The model under review builds one solid part; all positions refer to its coordinate system, in mm. Coordinates: 2 decimals unless noted, no trailing zeros. Loops run counter-clockwise (first coordinate to the right, second up) from the corner with the lowest first, then second, coordinate; pieces in that order, holes last. Notation, with made-up numbers: M 11.5,-16 L 15.5,-16 A16 ccw 15.5,10 Z; hole C 52.25,-17 d10. An arc over 180 degrees is marked long. Use one line per item in the form item = value.
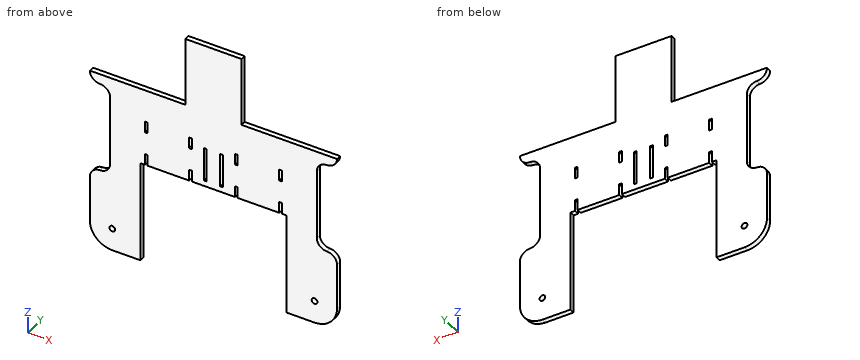
```python
from build123d import *

# Parameters (mm, degrees)
SKETCH1_W           = 279.4
SKETCH1_H           = 279.4
BOSS_EXTRUDE1_DEPTH = 5.715
CUT_EXTRUDE2_REACH  = 199.648
SKETCH4_W           = 22.86
SKETCH4_H           = 101.6
FILLET1_START       = -1
FILLET1_DEPTH       = 8
FILLET1_2_DEPTH     = 5.715
CUT_EXTRUDE3_REACH  = 199.648
SKETCH5_W           = 3.0988
SKETCH5_H           = 12.7
CUT_EXTRUDE4_REACH  = 199.648
SKETCH6_R           = 3.2639
FILLET2_R           = 25.4
CUT_EXTRUDE5_REACH  = 199.648
SKETCH7_W           = 165.1
SKETCH7_H           = 114.3
CUT_EXTRUDE7_REACH  = 199.648
SKETCH16_W          = 3.0988
SKETCH16_H          = 38.1
CUT_EXTRUDE11_REACH = 199.648
SKETCH26_W          = 107.95
SKETCH26_H          = 77.47


with BuildPart() as part:
    # Sketch1 → Boss-Extrude1 (new body)
    with BuildSketch(Plane(origin=(0, 0, 0), x_dir=(1, 0, 0), z_dir=(0, 1, 0))):
        Rectangle(SKETCH1_W, SKETCH1_H)
    extrude(amount=BOSS_EXTRUDE1_DEPTH)

    # Sketch4 → Cut-Extrude2 (cut, up to next)
    with BuildSketch(Plane(origin=(0, 5.715, 0), x_dir=(1, 0, 0), z_dir=(0, 1, 0)), mode=Mode.PRIVATE) as cut_extrude2_sk1:
        with Locations((-128.27, 0)):
            Rectangle(SKETCH4_W, SKETCH4_H)
    cut_extrude2_tool1 = extrude(cut_extrude2_sk1.sketch, amount=-CUT_EXTRUDE2_REACH, mode=Mode.PRIVATE) & part.part
    # Sketch4 → Cut-Extrude2 (cut, up to next)
    with BuildSketch(Plane(origin=(0, 5.715, 0), x_dir=(1, 0, 0), z_dir=(0, 1, 0)), mode=Mode.PRIVATE) as cut_extrude2_sk2:
        with Locations((128.27, 0)):
            Rectangle(SKETCH4_W, SKETCH4_H)
    cut_extrude2_tool2 = extrude(cut_extrude2_sk2.sketch, amount=-CUT_EXTRUDE2_REACH, mode=Mode.PRIVATE) & part.part
    add(cut_extrude2_tool1.solids().sort_by_distance((-128.27, 5.715, 0))[0], mode=Mode.SUBTRACT)
    add(cut_extrude2_tool2.solids().sort_by_distance((128.27, 5.715, 0))[0], mode=Mode.SUBTRACT)

    # Fillet1: read off the stored shape, not the designer's step
    # Fillet1 outline → Fillet1 (cut)
    with BuildSketch(Plane(origin=(0, 0, 0), x_dir=(1, 0, 0), z_dir=(0, 1, 0)).offset(FILLET1_START)):
        with BuildLine():
            ThreePointArc((-139.7, -62.23), (-136.352230509, -54.147769491), (-128.27, -50.8))
            Line((-128.27, -50.8), (-139.7, -50.8))
            Line((-139.7, -50.8), (-139.7, -62.23))
        make_face()
        with BuildLine():
            ThreePointArc((-128.27, 50.8), (-136.352230509, 54.147769491), (-139.7, 62.23))
            Line((-139.7, 62.23), (-139.7, 50.8))
            Line((-139.7, 50.8), (-128.27, 50.8))
        make_face()
        with BuildLine():
            Line((139.7, -50.8), (128.27, -50.8))
            ThreePointArc((128.27, -50.8), (136.352230509, -54.147769491), (139.7, -62.23))
            Line((139.7, -62.23), (139.7, -50.8))
        make_face()
        with BuildLine():
            ThreePointArc((139.7, 62.23), (136.352230509, 54.147769491), (128.27, 50.8))
            Line((128.27, 50.8), (139.7, 50.8))
            Line((139.7, 50.8), (139.7, 62.23))
        make_face()
    extrude(amount=FILLET1_DEPTH, mode=Mode.SUBTRACT)

    # Fillet1 2 outline → Fillet1 2 (add)
    with BuildSketch(Plane(origin=(0, 0, 0), x_dir=(1, 0, 0), z_dir=(0, 1, 0))):
        with BuildLine():
            Line((-116.84, -50.8), (-116.84, -39.37))
            ThreePointArc((-116.84, -39.37), (-120.187769491, -47.452230509), (-128.27, -50.8))
            Line((-128.27, -50.8), (-116.84, -50.8))
        make_face()
        with BuildLine():
            Line((-116.84, 50.8), (-128.27, 50.8))
            ThreePointArc((-128.27, 50.8), (-120.187769491, 47.452230509), (-116.84, 39.37))
            Line((-116.84, 39.37), (-116.84, 50.8))
        make_face()
        with BuildLine():
            Line((116.84, -50.8), (128.27, -50.8))
            ThreePointArc((128.27, -50.8), (120.187769491, -47.452230509), (116.84, -39.37))
            Line((116.84, -39.37), (116.84, -50.8))
        make_face()
        with BuildLine():
            Line((116.84, 50.8), (116.84, 39.37))
            ThreePointArc((116.84, 39.37), (120.187769491, 47.452230509), (128.27, 50.8))
            Line((128.27, 50.8), (116.84, 50.8))
        make_face()
    extrude(amount=FILLET1_2_DEPTH)

    # Sketch5 → Cut-Extrude3 (cut, up to next)
    with BuildSketch(Plane(origin=(0, 0, 0), x_dir=(-1, 0, 0), z_dir=(0, -1, 0)), mode=Mode.PRIVATE) as cut_extrude3_sk1:
        with Locations((75.8825, -19.05)):
            Rectangle(SKETCH5_W, SKETCH5_H)
    cut_extrude3_tool1 = extrude(cut_extrude3_sk1.sketch, amount=-CUT_EXTRUDE3_REACH, mode=Mode.PRIVATE) & part.part
    # Sketch5 → Cut-Extrude3 (cut, up to next)
    with BuildSketch(Plane(origin=(0, 0, 0), x_dir=(-1, 0, 0), z_dir=(0, -1, 0)), mode=Mode.PRIVATE) as cut_extrude3_sk2:
        with Locations((75.8825, 19.05)):
            Rectangle(SKETCH5_W, SKETCH5_H)
    cut_extrude3_tool2 = extrude(cut_extrude3_sk2.sketch, amount=-CUT_EXTRUDE3_REACH, mode=Mode.PRIVATE) & part.part
    # Sketch5 → Cut-Extrude3 (cut, up to next)
    with BuildSketch(Plane(origin=(0, 0, 0), x_dir=(-1, 0, 0), z_dir=(0, -1, 0)), mode=Mode.PRIVATE) as cut_extrude3_sk3:
        with Locations((-75.8825, 19.05)):
            Rectangle(SKETCH5_W, SKETCH5_H)
    cut_extrude3_tool3 = extrude(cut_extrude3_sk3.sketch, amount=-CUT_EXTRUDE3_REACH, mode=Mode.PRIVATE) & part.part
    # Sketch5 → Cut-Extrude3 (cut, up to next)
    with BuildSketch(Plane(origin=(0, 0, 0), x_dir=(-1, 0, 0), z_dir=(0, -1, 0)), mode=Mode.PRIVATE) as cut_extrude3_sk4:
        with Locations((-75.8825, -19.05)):
            Rectangle(SKETCH5_W, SKETCH5_H)
    cut_extrude3_tool4 = extrude(cut_extrude3_sk4.sketch, amount=-CUT_EXTRUDE3_REACH, mode=Mode.PRIVATE) & part.part
    # Sketch5 → Cut-Extrude3 (cut, up to next)
    with BuildSketch(Plane(origin=(0, 0, 0), x_dir=(-1, 0, 0), z_dir=(0, -1, 0)), mode=Mode.PRIVATE) as cut_extrude3_sk5:
        with Locations((25.908, -19.05)):
            Rectangle(SKETCH5_W, SKETCH5_H)
    cut_extrude3_tool5 = extrude(cut_extrude3_sk5.sketch, amount=-CUT_EXTRUDE3_REACH, mode=Mode.PRIVATE) & part.part
    # Sketch5 → Cut-Extrude3 (cut, up to next)
    with BuildSketch(Plane(origin=(0, 0, 0), x_dir=(-1, 0, 0), z_dir=(0, -1, 0)), mode=Mode.PRIVATE) as cut_extrude3_sk6:
        with Locations((25.908, 19.05)):
            Rectangle(SKETCH5_W, SKETCH5_H)
    cut_extrude3_tool6 = extrude(cut_extrude3_sk6.sketch, amount=-CUT_EXTRUDE3_REACH, mode=Mode.PRIVATE) & part.part
    # Sketch5 → Cut-Extrude3 (cut, up to next)
    with BuildSketch(Plane(origin=(0, 0, 0), x_dir=(-1, 0, 0), z_dir=(0, -1, 0)), mode=Mode.PRIVATE) as cut_extrude3_sk7:
        with Locations((-25.908, 19.05)):
            Rectangle(SKETCH5_W, SKETCH5_H)
    cut_extrude3_tool7 = extrude(cut_extrude3_sk7.sketch, amount=-CUT_EXTRUDE3_REACH, mode=Mode.PRIVATE) & part.part
    # Sketch5 → Cut-Extrude3 (cut, up to next)
    with BuildSketch(Plane(origin=(0, 0, 0), x_dir=(-1, 0, 0), z_dir=(0, -1, 0)), mode=Mode.PRIVATE) as cut_extrude3_sk8:
        with Locations((-25.908, -19.05)):
            Rectangle(SKETCH5_W, SKETCH5_H)
    cut_extrude3_tool8 = extrude(cut_extrude3_sk8.sketch, amount=-CUT_EXTRUDE3_REACH, mode=Mode.PRIVATE) & part.part
    add(cut_extrude3_tool1.solids().sort_by_distance((-75.8825, 0, 19.05))[0], mode=Mode.SUBTRACT)
    add(cut_extrude3_tool2.solids().sort_by_distance((-75.8825, 0, -19.05))[0], mode=Mode.SUBTRACT)
    add(cut_extrude3_tool3.solids().sort_by_distance((75.8825, 0, -19.05))[0], mode=Mode.SUBTRACT)
    add(cut_extrude3_tool4.solids().sort_by_distance((75.8825, 0, 19.05))[0], mode=Mode.SUBTRACT)
    add(cut_extrude3_tool5.solids().sort_by_distance((-25.908, 0, 19.05))[0], mode=Mode.SUBTRACT)
    add(cut_extrude3_tool6.solids().sort_by_distance((-25.908, 0, -19.05))[0], mode=Mode.SUBTRACT)
    add(cut_extrude3_tool7.solids().sort_by_distance((25.908, 0, -19.05))[0], mode=Mode.SUBTRACT)
    add(cut_extrude3_tool8.solids().sort_by_distance((25.908, 0, 19.05))[0], mode=Mode.SUBTRACT)

    # Sketch6 → Cut-Extrude4 (cut, up to next)
    with BuildSketch(Plane(origin=(0, 5.715, 0), x_dir=(1, 0, 0), z_dir=(0, 1, 0)), mode=Mode.PRIVATE) as cut_extrude4_sk1:
        with Locations(Location((-114.3, 114.3, 0), (0, 0, 270))):
            Circle(SKETCH6_R)
    cut_extrude4_tool1 = extrude(cut_extrude4_sk1.sketch, amount=-CUT_EXTRUDE4_REACH, mode=Mode.PRIVATE) & part.part
    # Sketch6 → Cut-Extrude4 (cut, up to next)
    with BuildSketch(Plane(origin=(0, 5.715, 0), x_dir=(1, 0, 0), z_dir=(0, 1, 0)), mode=Mode.PRIVATE) as cut_extrude4_sk2:
        with Locations(Location((114.3, 114.3, 0), (0, 0, 270))):
            Circle(SKETCH6_R)
    cut_extrude4_tool2 = extrude(cut_extrude4_sk2.sketch, amount=-CUT_EXTRUDE4_REACH, mode=Mode.PRIVATE) & part.part
    # Sketch6 → Cut-Extrude4 (cut, up to next)
    with BuildSketch(Plane(origin=(0, 5.715, 0), x_dir=(1, 0, 0), z_dir=(0, 1, 0)), mode=Mode.PRIVATE) as cut_extrude4_sk3:
        with Locations(Location((114.3, -114.3, 0), (0, 0, 270))):
            Circle(SKETCH6_R)
    cut_extrude4_tool3 = extrude(cut_extrude4_sk3.sketch, amount=-CUT_EXTRUDE4_REACH, mode=Mode.PRIVATE) & part.part
    # Sketch6 → Cut-Extrude4 (cut, up to next)
    with BuildSketch(Plane(origin=(0, 5.715, 0), x_dir=(1, 0, 0), z_dir=(0, 1, 0)), mode=Mode.PRIVATE) as cut_extrude4_sk4:
        with Locations(Location((-114.3, -114.3, 0), (0, 0, 270))):
            Circle(SKETCH6_R)
    cut_extrude4_tool4 = extrude(cut_extrude4_sk4.sketch, amount=-CUT_EXTRUDE4_REACH, mode=Mode.PRIVATE) & part.part
    add(cut_extrude4_tool1.solids().sort_by_distance((-114.3, 5.715, -114.3))[0], mode=Mode.SUBTRACT)
    add(cut_extrude4_tool2.solids().sort_by_distance((114.3, 5.715, -114.3))[0], mode=Mode.SUBTRACT)
    add(cut_extrude4_tool3.solids().sort_by_distance((114.3, 5.715, 114.3))[0], mode=Mode.SUBTRACT)
    add(cut_extrude4_tool4.solids().sort_by_distance((-114.3, 5.715, 114.3))[0], mode=Mode.SUBTRACT)

    # Fillet2
    fillet2_edges = [part.edges().sort_by_distance(p)[0] for p in [
        (-139.7, 2.8575, -139.7),
        (139.7, 2.8575, -139.7),
        (139.7, 2.8575, 139.7),
        (-139.7, 2.8575, 139.7),
    ]]
    fillet(fillet2_edges, radius=FILLET2_R)

    # Sketch7 → Cut-Extrude5 (cut, up to next)
    with BuildSketch(Plane(origin=(0, 5.715, 0), x_dir=(1, 0, 0), z_dir=(0, 1, 0)), mode=Mode.PRIVATE) as cut_extrude5_sk1:
        with Locations((0, 82.55)):
            Rectangle(SKETCH7_W, SKETCH7_H)
    cut_extrude5_tool1 = extrude(cut_extrude5_sk1.sketch, amount=-CUT_EXTRUDE5_REACH, mode=Mode.PRIVATE) & part.part
    add(cut_extrude5_tool1.solids().sort_by_distance((0, 5.715, -82.55))[0], mode=Mode.SUBTRACT)

    # Sketch16 → Cut-Extrude7 (cut, up to next)
    with BuildSketch(Plane(origin=(0, 5.715, 0), x_dir=(1, 0, 0), z_dir=(0, 1, 0)), mode=Mode.PRIVATE) as cut_extrude7_sk1:
        with Locations((-9.1948, 0)):
            Rectangle(SKETCH16_W, SKETCH16_H)
    cut_extrude7_tool1 = extrude(cut_extrude7_sk1.sketch, amount=-CUT_EXTRUDE7_REACH, mode=Mode.PRIVATE) & part.part
    # Sketch16 → Cut-Extrude7 (cut, up to next)
    with BuildSketch(Plane(origin=(0, 5.715, 0), x_dir=(1, 0, 0), z_dir=(0, 1, 0)), mode=Mode.PRIVATE) as cut_extrude7_sk2:
        with Locations((9.1948, 0)):
            Rectangle(SKETCH16_W, SKETCH16_H)
    cut_extrude7_tool2 = extrude(cut_extrude7_sk2.sketch, amount=-CUT_EXTRUDE7_REACH, mode=Mode.PRIVATE) & part.part
    add(cut_extrude7_tool1.solids().sort_by_distance((-9.1948, 5.715, 0))[0], mode=Mode.SUBTRACT)
    add(cut_extrude7_tool2.solids().sort_by_distance((9.1948, 5.715, 0))[0], mode=Mode.SUBTRACT)

    # Sketch26 → Cut-Extrude11 (cut, up to next)
    with BuildSketch(Plane(origin=(0, 5.715, 0), x_dir=(1, 0, 0), z_dir=(0, 1, 0)), mode=Mode.PRIVATE) as cut_extrude11_sk1:
        with Locations((-85.725, -100.965)):
            Rectangle(SKETCH26_W, SKETCH26_H)
    cut_extrude11_tool1 = extrude(cut_extrude11_sk1.sketch, amount=-CUT_EXTRUDE11_REACH, mode=Mode.PRIVATE) & part.part
    # Sketch26 → Cut-Extrude11 (cut, up to next)
    with BuildSketch(Plane(origin=(0, 5.715, 0), x_dir=(1, 0, 0), z_dir=(0, 1, 0)), mode=Mode.PRIVATE) as cut_extrude11_sk2:
        with Locations((85.725, -100.965)):
            Rectangle(SKETCH26_W, SKETCH26_H)
    cut_extrude11_tool2 = extrude(cut_extrude11_sk2.sketch, amount=-CUT_EXTRUDE11_REACH, mode=Mode.PRIVATE) & part.part
    add(cut_extrude11_tool1.solids().sort_by_distance((-85.725, 5.715, 100.965))[0], mode=Mode.SUBTRACT)
    add(cut_extrude11_tool2.solids().sort_by_distance((85.725, 5.715, 100.965))[0], mode=Mode.SUBTRACT)


solid = part.part
```
1. Add section D-D (z = 69). State the section outline as (x, y) points (3 decimals).
Response values:
outline = M -31.75,0 L 31.75,0 L 31.75,5.715 L -31.75,5.715 Z
2. Add section B-B (x = 14). State the section outline as (y, z) points (3 decimals), then the cut area to 3 significant figures.
Response values:
outline = M 0,-25.4 L 5.715,-25.4 L 5.715,139.7 L 0,139.7 Z
area = 944 mm^2
3. Insertion check: P1, Ø1.5, axis at x = -75, y = 5, coming from the +Z side; P2, Ø2.5, axis at x = 76, y = 3, coming from the -Z side; P3, Ø3, axis at y = 3, z = 93, coming from the -X side; P4, Ø5, axis at x = -114.3, z = -114.3, coming from the +Y side. Each pin has a flat end and moves straight along its axis. Give the tip position at first contact, or say it passes through.
Response values:
P1 = 62.23
P2 = -12.7
P3 = -31.75
P4 = through
4. Add section C-C (y = 3.3). Count the separate pieces of the cut face and the enclosed holes in it, then the cut area to 3 significant figures.
Response values:
separate_pieces = 1
enclosed_holes = 8
area = 36,900 mm^2
5. Add section A-A (z = -81.5). State the section outline as (x, y) points (3 decimals), then the cut area to 3 significant figures.
Response values:
outline = M -139.7,0 L -82.55,0 L -82.55,5.715 L -139.7,5.715 Z; M 82.55,0 L 139.7,0 L 139.7,5.715 L 82.55,5.715 Z
area = 653 mm^2
6. Wall thickness on line 1 along X through (y, z) = (4.7, 2); line 2 along X through (y, z) = (2.45, -114.3); line 3 along Z through (x, y) = (24.5, 5.3): over which ranges is each line inside the solid? List them lowest first. Write a range as from..to.
Response values:
line_1 = -116.84..-10.74, -7.65..7.65, 10.74..116.84
line_2 = -139.7..-117.56, -111.04..-82.55, 82.55..111.04, 117.56..139.7
line_3 = -12.7..12.7, 25.4..139.7
